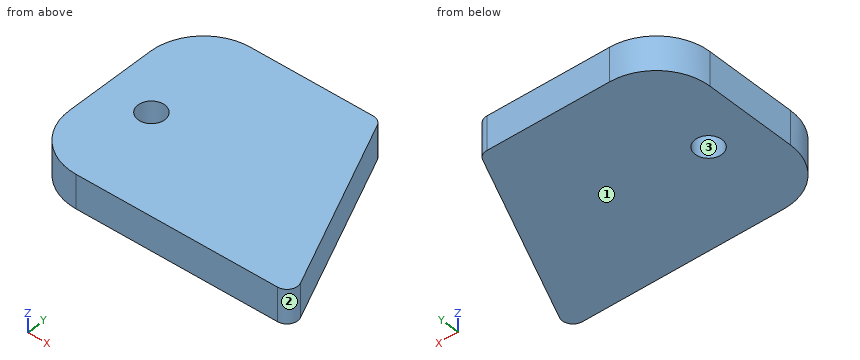
from build123d import *

# Parameters (mm, degrees)
BOSS_EXTRUDE1_DEPTH = 1.5875
FILLET1_R           = 1
FILLET2_R           = 5
SKETCH2_R           = 1.25
CUT_EXTRUDE1_DEPTH  = 17.357137005


with BuildPart() as part:
    # Sketch1 → Boss-Extrude1 (new, symmetric)
    with BuildSketch(Plane.XY):
        Polygon((-11.81540086, 9.32089354), (-11.81540086, -9.32089354), (12.941517766, -9.32089354), (13.597976447, -9.32089354), (5.339733299, 9.32089354), (4.683274618, 9.32089354), align=None)
    extrude(amount=BOSS_EXTRUDE1_DEPTH, both=True)

    # Fillet1
    fillet1_edges = [part.edges().sort_by_distance(p)[0] for p in [
        (5.339733299, 9.32089354, 0),
        (13.597976447, -9.32089354, 0),
    ]]
    fillet(fillet1_edges, radius=FILLET1_R)

    # Fillet2
    fillet2_edges = [part.edges().sort_by_distance(p)[0] for p in [
        (-11.81540086, -9.32089354, 0),
        (-11.81540086, 9.32089354, 0),
    ]]
    fillet(fillet2_edges, radius=FILLET2_R)

    # Sketch2 → Cut-Extrude1 (cut, through all)
    with BuildSketch(Plane.XY.offset(1.5875)):
        with Locations((-7.3274835, -0.67910646)):
            Circle(SKETCH2_R)
    extrude(amount=-CUT_EXTRUDE1_DEPTH, mode=Mode.SUBTRACT)


solid = part.part
Verification items for the finished model (mm, model axes). Face numbers are marked on the shaded views. Coordinates: 2 decimals unless noted, no trailing zeros. Write each loop counter-clockwise with the first axis right and the second up, starting at its lowest first coordinate (ties: lowest second). Pieces come first, ordered by that corner, then holes. Notation, with made-up numbers: M -34.75,61 L -22.75,61 A12 cw -22.75,76 Z; hole C 46,-23 d3. An arc over 180 degrees is marked long. Use CSV: the item, a comma, the result in double quotes.
Q1. Go/stop test with flat-tipped pins: P1, Ø1.5, axis at y = 6, z = 0, coming from the -X side; P2, Ø1, axis at y = -4, z = -0.5, coming from the +X side; P3, Ø2, axis at x = -7.33, y = -0.68, coming from the -Z side. Record where each tip stops, or that it passes through.
Computed values:
P1,"x = -11.73"
P2,"x = 11.46"
P3,"through"
Q2. Section check B-B, the plane y = -1. Enter the section's corners in (x, z).
Computed values:
outline,"M -11.82,-1.59 L -8.54,-1.59 L -8.54,1.59 L -11.82,1.59 Z; M -6.12,-1.59 L 9.91,-1.59 L 9.91,1.59 L -6.12,1.59 Z"
Q3. Mould release check, pull along Y, two halves, no side actions. Record for the marked faces 1, 2 and 3: pulls with the +Y half, pulls with the -Y half, needs draft (parallel to the pull), parting line crosses it, or undercut.
Computed values:
face 1,"needs draft"
face 2,"parting line crosses it"
face 3,"undercut"
Q4. Thickness scan on line 1 along Y through (x, z) = (-7.5, 1.35); line 2 along Y through (x, z) = (-8.25, -1.4); line 3 along X through (y, z) = (4.75, 0.25). Record the ranges inside material, lowest first. Write a range as [from, to].
Computed values:
line 1,"[-9.27, -1.92], [0.56, 9.27]"
line 2,"[-9.11, -1.52], [0.16, 9.11]"
line 3,"[-11.8, 7.36]"
Q5. Section check C-C, the plane x = -10. Enter the section's corners in (y, z), and give its area (3 significant figures).
Computed values:
outline,"M -8.18,-1.59 L 8.18,-1.59 L 8.18,1.59 L -8.18,1.59 Z"
area,"51.9 mm²"
Q6. Section check D-D, the plane y = 3.5. Enter the section's corners in (x, z), and give its area (3 significant figures).
Computed values:
outline,"M -11.82,-1.59 L 7.92,-1.59 L 7.92,1.59 L -11.82,1.59 Z"
area,"62.7 mm²"
Q7. Section check A-A, the plane z = 0.55. Enter the section's corners in (x, y), and give its area (3 significant figures).
Computed values:
outline,"M -11.82,-4.32 A5 ccw -6.82,-9.32 L 12.06,-9.32 A1 ccw 12.98,-7.92 L 5.6,8.73 A1 ccw 4.69,9.32 L -6.82,9.32 A5 ccw -11.82,4.32 Z; hole C -7.33,-0.68 d2.5"
area,"381 mm²"
